Geometry check sheet. Reference: the model listing, model coordinates, mm. Face numbers are marked on the shaded views. A direction names the side the tool comes from. Round coordinates to 2 decimals unless told otherwise and drop trailing zeros. Loops run counter-clockwise (first coordinate to the right, second up) from the corner with the lowest first, then second, coordinate; pieces in that order, holes last. Notation, with made-up numbers: (17.25, -39.5) - (68.25, -39.5) arc R35 ccw to (68.25, -3.5) - close; hole circle Ø3 at (-7.5, 87.5). An arc over 180 degrees is marked (long way). Answer as CSV lines item,"result". Start each with the question number.
1) Cross-section at C-C on y = -130.5. Record the boundary of the cut face in (x, z).
2) Cross-section at D-D on y = -25. Record the boundary of the cut face in (x, z).
3) Cross-section at A-A on z = 0. State how many separate pieces and enclosed holes the cut face has, and give its area (3 significant figures).
4) Cross-section at B-B on x = 0. Record the boundary of the cut face in (y, z), and give its area (3 significant figures).
5) Access from +Z, -Z, +X, -X, +Y, -Y to the whole of each face (thin tool, end or side, straight path). Record for the marked faces 5 and 6.
6) Draft check along Z on the marked faces 1, 2, 3 and 4. Enter one of: released by +Z, released by -Z, zero draft, split by the parting line, or undercut.
7) Depth check by flat-ended pin: P1, Ø10, axis at y = -257.5, z = 229, coming from the +X side; P2, Ø6, axis at y = 200, z = 135, coming from the -X side; P3, Ø1.5, axis at x = -216, y = 302, coming from the +Z side. Enter the tip coordinate at first touch or a pass-through.
8) Thickness scan on line 1 along Y through (x, z) = (-265, -307); line 2 along Y through (x, z) = (-368, 0); line 3 along Y through (x, z) = (300, 165.5). Record the ranges inside material, lowest first.
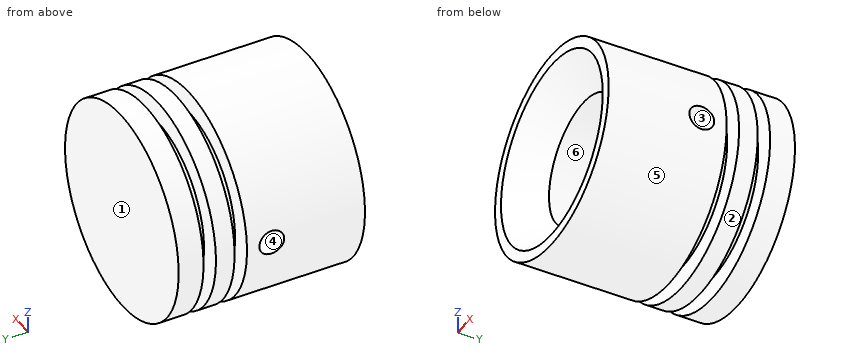
from build123d import *

# Parameters (mm, degrees)
CUT_EXTRUDE1_DEPTH      = 713.163187058
CUT_EXTRUDE1_DEPTH_BACK = 713.163187058
SKETCH4_R               = 50.8


with BuildPart() as part:
    # Sketch3 → Revolve1 (revolve)
    with BuildSketch(Plane.XY, mode=Mode.PRIVATE) as revolve1_sk:
        Polygon((0, 381), (0, 304.8), (-254, 304.8), (-254, -254), (-381, -381), (-425.45, -381), (-425.45, 101.6), (-336.55, 101.6), (-336.55, 152.4), (-425.45, 152.4), (-425.45, 228.6), (-336.55, 228.6), (-336.55, 279.4), (-425.45, 279.4), (-425.45, 381), align=None)
    revolve(revolve1_sk.sketch.rotate(Axis((0, -381, 0), (0, 1, 0)), 270), axis=Axis((0, -381, 0), (0, 1, 0)))

    # Sketch4 → Cut-Extrude1 (cut, two sides: drawn at the far end of the back side and taken through both)
    with BuildSketch(Plane(origin=(0, 0, 0), x_dir=(0, 0, -1), z_dir=(1, 0, 0)).offset(-CUT_EXTRUDE1_DEPTH_BACK)):
        Circle(SKETCH4_R)
    extrude(amount=CUT_EXTRUDE1_DEPTH + CUT_EXTRUDE1_DEPTH_BACK, mode=Mode.SUBTRACT)


solid = part.part
Answer block:
1,outline,"circle Ø850.9 at (0, 0); hole circle Ø508 at (0, 0)"
2,outline,"(-423.15, -44.22) arc R425.45 ccw to (423.15, -44.22) - (250.12, -44.22) arc R254 cw to (-250.12, -44.22) - close; (-423.15, 44.22) - (-250.12, 44.22) arc R254 cw to (250.12, 44.22) - (423.15, 44.22) arc R425.45 ccw to start"
3,separate pieces,"3"
3,enclosed holes,"0"
3,area,"231,000 mm^2"
4,outline,"(-381, -425.45) - (101.6, -425.45) - (101.6, -336.55) - (152.4, -336.55) - (152.4, -425.45) - (228.6, -425.45) - (228.6, -336.55) - (279.4, -336.55) - (279.4, -425.45) - (381, -425.45) - (381, 425.45) - (279.4, 425.45) - (279.4, 336.55) - (228.6, 336.55) - (228.6, 425.45) - (152.4, 425.45) - (152.4, 336.55) - (101.6, 336.55) - (101.6, 425.45) - (-381, 425.45) - (-381, 381) - (-254, 254) - (304.8, 254) - (304.8, -254) - (-254, -254) - (-381, -381) - close"
4,area,"266,000 mm^2"
5,face 5,"+Y, -Y"
5,face 6,"-Y"
6,face 1,"zero draft"
6,face 2,"split by the parting line"
6,face 3,"undercut"
6,face 4,"undercut"
7,P1,"stops at x = 361.71"
7,P2,"stops at x = -404.45"
7,P3,"stops at z = 366.98"
8,line 1,"y = -381 to 101.6, 152.4 to 228.6, 279.4 to 381"
8,line 2,"y = -368 to -50.8, 50.8 to 101.6, 152.4 to 228.6, 279.4 to 381"
8,line 3,"y = -342.62 to 101.6, 152.4 to 228.6, 279.4 to 381"
